Check sheet for the modelled part. Datum: model origin and axes. Units: mm. Face numbers are marked on the shaded views. Give positions to 0.01 mm unless a question says otherwise; leave off trailing zeros. Write each loop counter-clockwise with the first axis right and the second up, starting at its lowest first coordinate (ties: lowest second). Pieces come first, ordered by that corner, then holes. Notation, with made-up numbers: M 80.25,73 L 130.25,73 A31 ccw 130.25,97 Z; hole C 40,40.5 d9. An arc over 180 degrees is marked long. Write item = value, one per line. Start each with the question number.
1) Go/stop test with flat-tipped pins: pin 1 (0.7 mm diameter, centred on x = -4, y = 0.5, fed in from -Z); pin 2 (1.1 mm diameter, centred on y = 0.5, z = 1.5, fed in from -X); pin 3 (4 mm diameter, centred on x = 29.5, y = 0, fed in from +Z); pin 4 (4 mm diameter, centred on x = 27, z = -2, fed in from +Y). Record where each tip stops, or that it passes through.
2) Scan lines: line 1 along Y through (x, z) = (28, 1.5); line 2 along X through (y, z) = (0.5, 3.25); line 3 along Z through (x, y) = (28, 0). Record each from-to range of solid material in increasing order. Write a range as [from, to].
3) Cross-section at A-A, the plane x = 41. Record the cut outline in (y, z), plus the area to 3 significant figures.
4) Mould release check, pull along Z, two halves, no side actions. Record for the marked faces 1, 2 and 3: released by +Z, released by -Z, zero draft, split by the parting line, or undercut.
Autodesk Inventor part; units mm, degrees
ref_plane "bolt_XY" through (0, 0, 0) normal (1, 0, 0) x (0, 0, -1)
ref_plane "bolt_YZ" through (0, 0, 0) normal (0, 0, -1) x (0, 1, 0)
ref_plane "bolt_ZX" through (0, 0, 0) normal (0, 1, 0) x (1, 0, 0)
sketch "Sketch_1" plane through (0, 0, 0) normal (0, 0, 1) x (1, 0, 0)
  line L0 (22, 0) -> (-5, 0)
  line L1 (-5, 0) -> (-5, 3.75)
  line L2 (-5, 3.75) -> (-4.5, 4.25)
  line L3 (-4.5, 4.25) -> (0, 4.25)
  line L4 (0, 4.25) -> (0, 2.5)
  line L5 (0, 2.5) -> (45.5095, 2.5)
  line L6 (45.5095, 2.5) -> (46, 2.0095)
  line L7 (46, 2.0095) -> (46, 0)
  line L8 (46, 0) -> (-5, 0)
  dimension "d14" = 45
  dimension "d16" = 45
  dimension "d17" = 4.5
  dimension "d18" = 3.75
  dimension "d19" = 2.0095
  dimension "d20" = 46
revolve "Revolution1" add sketch "Sketch_1" angle 360 about axis through (22, 0, 0) along (1, 0, 0)
thread "Thread1"
sketch "Sketch2" plane through (-5, 0, 0) normal (-1, 0, 0) x (0, 0, 1)
  point P0 (0, 0)
hole "Hole1" at (-5, 0, 0) direction (1, 0, 0) diameter 4 depth 2.5 tip angle 150
sketch "Sketch_3" plane through (-5, 0, 0) normal (1, 0, 0) x (0, 0, -1)
  line L0 (-2, -1.1547) -> (0, -2.3094)
  line L1 (0, -2.3094) -> (2, -1.1547)
  line L2 (2, -1.1547) -> (2, 1.1547)
  line L3 (2, 1.1547) -> (0, 2.3094)
  line L4 (0, 2.3094) -> (-2, 1.1547)
  line L5 (-2, 1.1547) -> (-2, -1.1547)
extrude "Extrusion1" cut sketch "Sketch_3" along normal blind 2.5
ref_plane "bolt_XY" through (0, 0, 0) normal (1, 0, 0) x (0, 0, -1)
ref_plane "bolt_YZ" through (0, 0, 0) normal (0, 0, -1) x (0, 1, 0)
ref_plane "bolt_ZX" through (0, 0, 0) normal (0, 1, 0) x (1, 0, 0)
ref_plane "nut_XY" through (22, 0, 0) normal (1, 0, 0) x (0, 0, -1)
ref_plane "nut_YZ" through (22, 0, 0) normal (0, 0, -1) x (0, 1, 0)
ref_plane "nut_ZX" through (22, 0, 0) normal (0, 1, 0) x (1, 0, 0)
properties part number "SCB5-46" material "鋼"
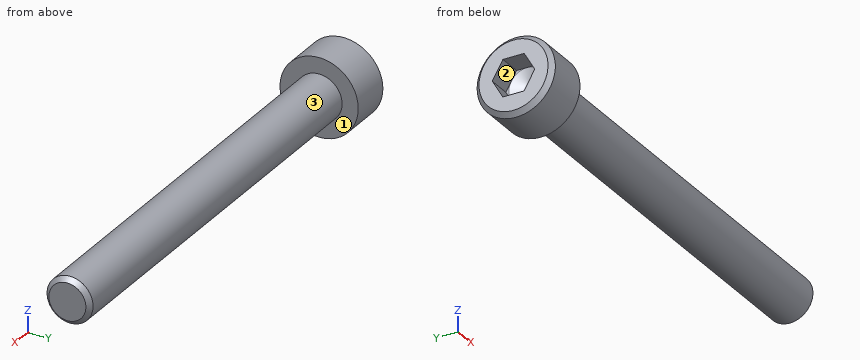
Reply:
q1.pin_1 = -4.25
q1.pin_2 = -5
q1.pin_3 = 2.5
q1.pin_4 = 2.5
q2.line_1 = [-2, 2]
q2.line_2 = [-5, 0]
q2.line_3 = [-2.5, 2.5]
q3.outline = C 0,0 d5
q3.area = 19.6 mm2
q4.face_1 = zero draft
q4.face_2 = undercut
q4.face_3 = split by the parting line
